from build123d import *

# Parameters (mm, degrees)
F0_R     = 2.5
F1_DEPTH = 5


with BuildPart() as f1:
    # F0 (on Top) → F1 (new body)
    with BuildSketch(Plane.XY):
        with BuildLine():
            Line((-35, -57.5), (35, -57.5))
            ThreePointArc((35, -57.5), (42.071068, -54.571068), (45, -47.5))
            Line((45, -47.5), (45, 43.5))
            ThreePointArc((45, 43.5), (42.071068, 50.571068), (35, 53.5))
            Line((35, 53.5), (30, 53.5))
            Line((30, 53.5), (30, 51.5))
            ThreePointArc((30, 51.5), (32.12132, 46.37868), (27, 48.5))
            Line((27, 48.5), (-27, 48.5))
            ThreePointArc((-27, 48.5), (-32.12132, 46.37868), (-30, 51.5))
            Line((-30, 51.5), (-30, 53.5))
            Line((-30, 53.5), (-35, 53.5))
            ThreePointArc((-35, 53.5), (-42.071068, 50.571068), (-45, 43.5))
            Line((-45, 43.5), (-45, -47.5))
            ThreePointArc((-45, -47.5), (-42.071068, -54.571068), (-35, -57.5))
        make_face()
        with Locations((-15, -42.5)):
            Circle(F0_R, mode=Mode.SUBTRACT)
        with Locations((-15, -10.5)):
            Circle(F0_R, mode=Mode.SUBTRACT)
        with Locations((15, -42.5)):
            Circle(F0_R, mode=Mode.SUBTRACT)
        with Locations((15, -10.5)):
            Circle(F0_R, mode=Mode.SUBTRACT)
    extrude(amount=F1_DEPTH)


solid = f1.part
Source: CAD feature listing. Evaluate the final solid. Frame: model axes, mm. A direction names the side the tool comes from. Coordinates: 2 decimals unless noted, no trailing zeros. Order: outer loops, then holes, each group sorted by start corner. A loop starts at its lowest first (then second) coordinate and runs counter-clockwise, first axis right, second up.
Item 1: Pull-direction query (X, two-part tool) for faces 3 (the face through (13, -12, 2)), 4 (the face through (45, -3, 2)), 5 (the face through (14.46, -44.94, 2.46)), 6 (the face through (33, 53.5, 2)); classes: pulls with the +X half, pulls with the -X half, needs draft (parallel to the pull), parting line crosses it, or undercut.
Output values:
face 3: undercut
face 4: pulls with the +X half
face 5: undercut
face 6: needs draft
Item 2: Cut plane B-B (y = -10.5). Return loops of the section in (x, z).
Output values:
outline: (-45, 0) - (-17.5, 0) - (-17.5, 5) - (-45, 5) - close; (-12.5, 0) - (12.5, 0) - (12.5, 5) - (-12.5, 5) - close; (17.5, 0) - (45, 0) - (45, 5) - (17.5, 5) - close
Item 3: Cut plane D-D (x = -3). Return loops of the section in (y, z).
Output values:
outline: (-57.5, 0) - (48.5, 0) - (48.5, 5) - (-57.5, 5) - close
Item 4: Material intervals for line 1 (Y direction, x = 15, z = 2.3); line 2 (X direction, y = -41.5, z = 2.4); line 3 (Y direction, x = 23.5, z = 3.65), sorted ascending.
Output values:
line 1: y = -57.5 to -45, -40 to -13, -8 to 48.5
line 2: x = -45 to -17.29, -12.71 to 12.71, 17.29 to 45
line 3: y = -57.5 to 48.5
Item 5: First-contact query: P1, Ø5.5, axis at x = -30, y = 48.5, coming from the -Z side; P2, Ø0.6, axis at y = 52.5, z = 1.5, coming from the -X side; P3, Ø2, axis at y = 53, z = 2, coming from the +X side; P4, Ø1.5, axis at x = 13, z = 3.5, coming from the +Y side. Flat tips, straight axial feed; report the tip coordinate or a pass-through.
Output values:
P1: passes through
P2: stops at x = -39.93
P3: stops at x = 40.27
P4: stops at y = 48.5
Item 6: Cut plane A-A (x = 15). Return loops of the section in (y, z), plus the area to 3 significant figures.
Output values:
outline: (-57.5, 0) - (-45, 0) - (-45, 5) - (-57.5, 5) - close; (-40, 0) - (-13, 0) - (-13, 5) - (-40, 5) - close; (-8, 0) - (48.5, 0) - (48.5, 5) - (-8, 5) - close
area: 480 mm2
Item 7: Cut plane C-C (z = 1.25). Return loops of the section in (x, y), plus the area to 3 significant figures.
Output values:
outline: (-45, -47.5) arc R10 ccw to (-35, -57.5) - (35, -57.5) arc R10 ccw to (45, -47.5) - (45, 43.5) arc R10 ccw to (35, 53.5) - (30, 53.5) - (30, 51.5) arc R3 cw (long way) to (27, 48.5) - (-27, 48.5) arc R3 cw (long way) to (-30, 51.5) - (-30, 53.5) - (-35, 53.5) arc R10 ccw to (-45, 43.5) - close; hole circle Ø5 at (-15, -42.5); hole circle Ø5 at (-15, -10.5); hole circle Ø5 at (15, -42.5); hole circle Ø5 at (15, -10.5)
area: 9,480 mm2
Item 8: Set-up query: faces 1 (the face through (-1, -1, 5)), 2 (the face through (0, 48.5, 2)). Return all of +Z, -Z, +X, -X, +Y, -Y with unobstructed straight access to the full face (end or side cutting, diameter ignored); none if empty.
Output values:
face 1: +Z, +X, -X, +Y, -Y
face 2: +Z, -Z, +Y
